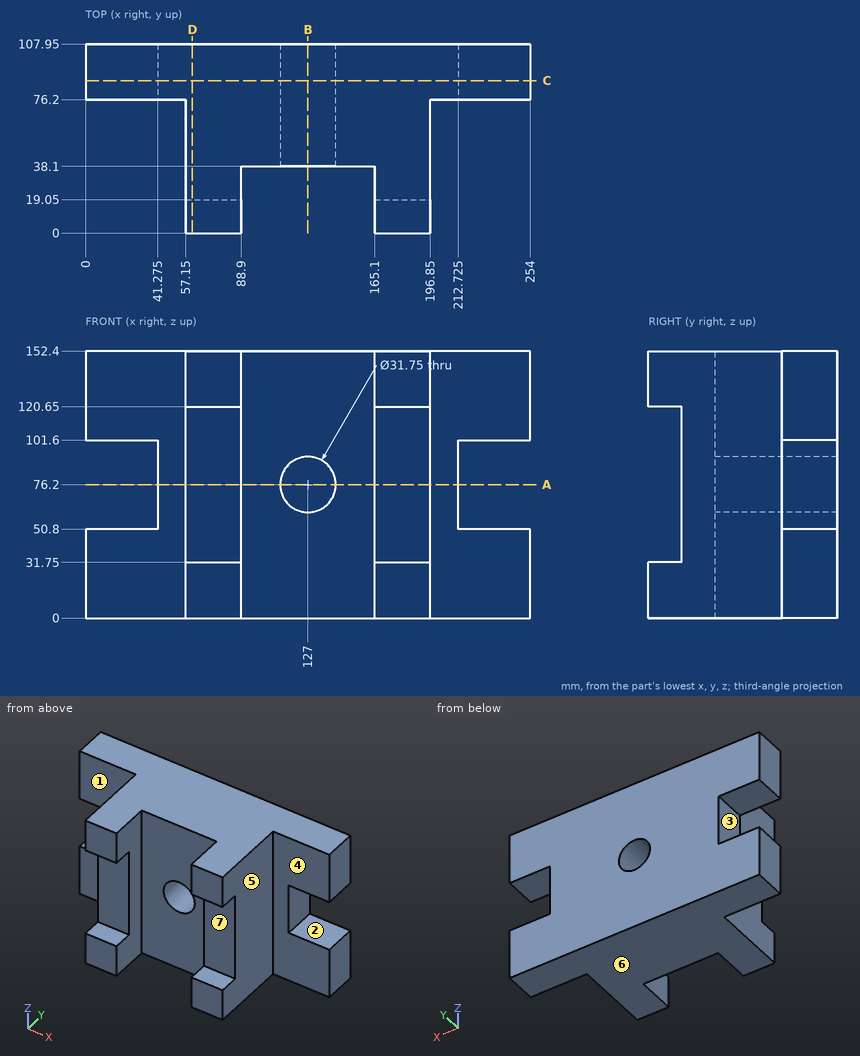
Part print with two shaded views. Sizes in mm from the minimum x, y, z corner. A direction names the side the tool comes from. Give positions to 0.01 mm unless a question says otherwise; leave off trailing zeros. Order: outer loops, then holes, each group sorted by start corner. A loop starts at its lowest first (then second) coordinate and runs counter-clockwise, first axis right, second up. Notation, with made-up numbers: (4.25, -22) - (57.25, -22) arc R13 cw to (57.25, -4) - close; hole circle Ø8 at (88.25, 34.5). An arc over 180 degrees is marked (long way). Write each question's results on one line, items separated by ' | '.
1. 3-axis set-ups, long thin cutter, end or side, ignore diameter. For the marked faces 1, 2, 3 and 4: which of +Z, -Z, +X, -X, +Y, -Y reach the whole face in a straight line?
Calculated:
face 1: +Z, -Z, -X, -Y | face 2: +X, +Y, -Y | face 3: -X, +Y, -Y | face 4: +Z, -Z, +X, -Y
2. Saw through at D-D on x = 61. List the corners of the cut face in (y, z), and give its area (3 significant figures).
Calculated:
outline: (0, 0) - (107.95, 0) - (107.95, 152.4) - (0, 152.4) - (0, 120.65) - (19.05, 120.65) - (19.05, 31.75) - (0, 31.75) - close | area: 14,800 mm2
3. Saw through at C-C on y = 87. List the corners of the cut face in (x, z) (3 decimals), and give its area (3 significant figures).
Calculated:
outline: (0, 0) - (254, 0) - (254, 50.8) - (212.725, 50.8) - (212.725, 101.6) - (254, 101.6) - (254, 152.4) - (0, 152.4) - (0, 101.6) - (41.275, 101.6) - (41.275, 50.8) - (0, 50.8) - close; hole circle Ø31.75 at (127, 76.2) | area: 33,700 mm2
4. Saw through at B-B on x = 127. List the corners of the cut face in (y, z) (3 decimals), and give its area (3 significant figures).
Calculated:
outline: (38.1, 0) - (107.95, 0) - (107.95, 60.325) - (38.1, 60.325) - close; (38.1, 92.075) - (107.95, 92.075) - (107.95, 152.4) - (38.1, 152.4) - close | area: 8,430 mm2
5. Pin check, flat tips, straight feed: pin 1 (16 mm diameter, centred on y = 86.5, z = 71, fed in from -X) (3 decimals); pin 2 (8 mm diameter, centred on y = 56.5, z = 68, fed in from +X); pin 3 (10 mm diameter, centred on x = 98, z = 24, fed in from -Y). Stop position of each tip, or through.
Calculated:
pin 1: stops at x = 41.275 | pin 2: stops at x = 196.85 | pin 3: stops at y = 38.1
6. Probe L1, parallel to Z at x = 127, y = 86 (3 decimals); L2, parallel to X at y = 79, z = 76 (3 decimals); L3, parallel to X at y = 61, z = 76. List the from-to ranges inside material, lowest first. Write a range as from..to.
Calculated:
L1: z = 0..60.325, 92.075..152.4 | L2: x = 41.275..111.126, 142.874..212.725 | L3: x = 57.15..111.13, 142.87..196.85
7. Saw through at A-A on z = 76.2. List the corners of the cut face in (x, y) (3 decimals), and give its area (3 significant figures).
Calculated:
outline: (41.275, 76.2) - (57.15, 76.2) - (57.15, 19.05) - (88.9, 19.05) - (88.9, 38.1) - (111.125, 38.1) - (111.125, 107.95) - (41.275, 107.95) - close; (142.875, 38.1) - (165.1, 38.1) - (165.1, 19.05) - (196.85, 19.05) - (196.85, 76.2) - (212.725, 76.2) - (212.725, 107.95) - (142.875, 107.95) - close | area: 9,760 mm2
8. Pull direction Z, two halves, no side cores. Call the marked faces 5, 6 and 7: released by +Z, released by -Z, zero draft, split by the parting line, or undercut.
Calculated:
face 5: zero draft | face 6: released by -Z | face 7: undercut
